from build123d import *

# Parameters (mm, degrees)
EXTRUDE1_DEPTH         = 12
M10_GEVINDHULLER_D     = 8.5
M10_GEVINDHULLER_DEPTH = 22
M10_GEVINDHULLER_TIP   = 2.553657631


with BuildPart() as part:
    # Sketch1 → Extrude1 (new body)
    with BuildSketch(Plane.XY):
        with BuildLine():
            Line((36.5, 3), (36.5, 8.529437252))
            ThreePointArc((36.5, 8.529437252), (37.41344561, 13.12163844), (40.014718626, 17.014718626))
            Line((40.014718626, 17.014718626), (64.485281374, 41.485281374))
            ThreePointArc((64.485281374, 41.485281374), (67.08655439, 45.37836156), (68, 49.970562748))
            Line((68, 49.970562748), (68, 68))
            ThreePointArc((68, 68), (66.611898825, 70.530174337), (63.732145215, 70.718923361))
            Line((63.732145215, 70.718923361), (8.939617358, 45.168748012))
            ThreePointArc((8.939617358, 45.168748012), (8.345295598, 44.801908517), (7.851901649, 44.307588803))
            ThreePointArc((7.851901649, 44.307588803), (0, 40.500135977), (-7.851901649, 44.307588803))
            ThreePointArc((-7.851901649, 44.307588803), (-8.345295598, 44.801908517), (-8.939617358, 45.168748012))
            Line((-8.939617358, 45.168748012), (-63.732145215, 70.718923361))
            ThreePointArc((-63.732145215, 70.718923361), (-66.611898825, 70.530174337), (-68, 68))
            Line((-68, 68), (-68, 49.970562748))
            ThreePointArc((-68, 49.970562748), (-67.08655439, 45.37836156), (-64.485281374, 41.485281374))
            Line((-64.485281374, 41.485281374), (-40.014718626, 17.014718626))
            ThreePointArc((-40.014718626, 17.014718626), (-37.41344561, 13.12163844), (-36.5, 8.529437252))
            Line((-36.5, 8.529437252), (-36.5, 3))
            ThreePointArc((-36.5, 3), (-35.621320344, 0.878679656), (-33.5, 0))
            Line((-33.5, 0), (0, 0))
            Line((0, 0), (33.5, 0))
            ThreePointArc((33.5, 0), (35.621320344, 0.878679656), (36.5, 3))
        make_face()
    extrude(amount=EXTRUDE1_DEPTH)

    # M10 gevindhuller
    with Locations(Plane.XY.offset(12)):
        with Locations((-36, 44.546676643), (0, 28.546676643), (36, 44.546676643)):
            Hole(M10_GEVINDHULLER_D / 2, depth=M10_GEVINDHULLER_DEPTH)
            with Locations((0, 0, -(M10_GEVINDHULLER_DEPTH + M10_GEVINDHULLER_TIP / 2))):  # 118° drill point
                Cone(0, M10_GEVINDHULLER_D / 2, M10_GEVINDHULLER_TIP, mode=Mode.SUBTRACT)


solid = part.part
Geometry check sheet. Reference: the model listing, model coordinates, mm. A direction names the side the tool comes from. Round coordinates to 2 decimals unless told otherwise and drop trailing zeros. Loops run counter-clockwise (first coordinate to the right, second up) from the corner with the lowest first, then second, coordinate; pieces in that order, holes last. Notation, with made-up numbers: (82, -23) -> (127, -23) arc R27 cw to (127, 12) -> close; hole circle Ø6 at (45.25, 3.25). An arc over 180 degrees is marked (long way). Answer as a JSON object with one key per item and string values. Group by question number.
Item 1: Release check for a two-part mould opening along X. For faces 5 (the face through (-32.6, 42, 5.9)), 6 (the face through (0, 0, 6)), 7 (the face through (-37.439, 13.183, 5.916)) record: pulls with the +X half, pulls with the -X half, needs draft (parallel to the pull), parting line crosses it, or undercut.
Item 2: Cross-section at C-C, the plane y = 5. Record the cut outline in (x, z), plus the area to 3 significant figures.
Item 3: Thickness scan on line 1 along X through (y, z) = (48, 9.75); line 2 along X through (y, z) = (43, 11.75); line 3 along X through (y, z) = (51.5, 11). Record the ranges inside material, lowest first.
Item 4: Cross-section at D-D, the plane x = -42. Record the cut outline in (y, z).
Item 5: Cross-section at B-B, the plane z = 7.5. Record the cut outline in (x, y), plus the area to 3 significant figures.
Item 6: Depth check by flat-ended pin: pin 1 Ø4 at (y, z) = (8, 5) entering from -X; pin 2 Ø6 at (y, z) = (29, 2.5) entering from +X; pin 3 Ø4.5 at (y, z) = (4.5, 8.5) entering from +X. Enter the tip coordinate at first touch or a pass-through.
Item 7: Cross-section at A-A, the plane x = 0. Record the cut outline in (y, z), plus the area to 3 significant figures.
Item 8: Set-up check for faces 1 (the face through (-68, 59, 6)), 2 (the face through (36.5, 6, 6)), 3 (the face through (-35.952, 57.765, 5.916)), 4 (the face through (-36.5, 6, 6)): record each of +Z, -Z, +X, -X, +Y, -Y from which the full face is reachable in a straight line by a thin tool's end or side.
Determined:
{
 "1": {"face 5": "undercut", "face 6": "needs draft", "face 7": "pulls with the -X half"},
 "2": {"outline": "(-36.5, 0) -> (36.5, 0) -> (36.5, 12) -> (-36.5, 12) -> close", "area": "876 mm²"},
 "3": {"line 1": "x = -67.84 to -38.48, -33.52 to -15.01, 15.01 to 33.52, 38.48 to 67.84", "line 2": "x = -65.77 to -39.96, -32.04 to -6.61, 6.61 to 32.04, 39.96 to 65.77", "line 3": "x = -68 to -22.52, 22.52 to 68"},
 "4": {"outline": "(19, 0) -> (60.59, 0) -> (60.59, 12) -> (19, 12) -> close"},
 "5": {"outline": "(-68, 49.97) arc R12 ccw to (-64.49, 41.49) -> (-40.01, 17.01) arc R12 cw to (-36.5, 8.53) -> (-36.5, 3) arc R3 ccw to (-33.5, 0) -> (33.5, 0) arc R3 ccw to (36.5, 3) -> (36.5, 8.53) arc R12 cw to (40.01, 17.01) -> (64.49, 41.49) arc R12 ccw to (68, 49.97) -> (68, 68) arc R3 ccw to (63.73, 70.72) -> (8.94, 45.17) arc R3 ccw to (7.85, 44.31) arc R10 cw to (-7.85, 44.31) arc R3 ccw to (-8.94, 45.17) -> (-63.73, 70.72) arc R3 ccw to (-68, 68) -> close; hole circle Ø8.5 at (-36, 44.55); hole circle Ø8.5 at (0, 28.55); hole circle Ø8.5 at (36, 44.55)", "area": "5,690 mm²"},
 "6": {"pin 1": "stops at x = -36.59", "pin 2": "stops at x = 55", "pin 3": "stops at x = 36.5"},
 "7": {"outline": "(0, 0) -> (24.3, 0) -> (24.3, 12) -> (0, 12) -> close; (32.8, 0) -> (40.5, 0) -> (40.5, 12) -> (32.8, 12) -> close", "area": "384 mm²"},
 "8": {"face 1": "+Z, -Z, -X, +Y, -Y", "face 2": "+Z, -Z, +X, -Y", "face 3": "+Z, -Z, +Y", "face 4": "+Z, -Z, -X, -Y"}
}
